Input: part model. Units: mm. Frame: model coordinates. A direction names the side the tool comes from. Give positions to 0.01 mm unless a question says otherwise; leave off trailing zeros. Write each loop counter-clockwise with the first axis right and the second up, starting at its lowest first coordinate (ties: lowest second). Pieces come first, ordered by that corner, then holes. Notation, with made-up numbers: (71.5, -30.5) -> (128.5, -30.5) arc R22 ccw to (128.5, -9.5) -> close; hole circle Ø6 at (-36.75, 5). An arc over 180 degrees is marked (long way). Answer as a JSON object with one key per item and string values. Group by question number.
from build123d import *

# Parameters (mm, degrees)
F0_R     = 0.8
F0_R_2   = 1.6
F0_R_3   = 1.2
F1_DEPTH = 4
F2_W     = 34.4678
F2_H     = 0.2
F3_DEPTH = 3.8


with BuildPart() as f1:
    # F0 (on Front) → F1 (new body)
    with BuildSketch(Plane.XZ):
        with BuildLine():
            Line((-76.973173, -27.461596), (-105.598973, -27.461596))
            ThreePointArc((-105.598973, -27.461596), (-107.664432, -28.317137), (-108.519973, -30.382596))
            Line((-108.519973, -30.382596), (-108.519973, -48.797596))
            ThreePointArc((-108.519973, -48.797596), (-107.664432, -50.863055), (-105.598973, -51.718596))
            Line((-105.598973, -51.718596), (-76.973173, -51.718596))
            ThreePointArc((-76.973173, -51.718596), (-74.907714, -50.863055), (-74.052173, -48.797596))
            Line((-74.052173, -48.797596), (-74.052173, -30.382596))
            ThreePointArc((-74.052173, -30.382596), (-74.907714, -28.317137), (-76.973173, -27.461596))
        make_face()
        with Locations((-102.017573, -45.266996)):
            Circle(F0_R, mode=Mode.SUBTRACT)
        with Locations((-97.648773, -45.266996)):
            Circle(F0_R, mode=Mode.SUBTRACT)
        with Locations((-93.279973, -45.266996)):
            Circle(F0_R, mode=Mode.SUBTRACT)
        with Locations((-99.833173, -41.482396)):
            Circle(F0_R, mode=Mode.SUBTRACT)
        with Locations((-95.464373, -41.482396)):
            Circle(F0_R, mode=Mode.SUBTRACT)
        with BuildLine():
            ThreePointArc((-77.666642, -47.210096), (-76.839663, -45.530643), (-75.379473, -46.702096))
            ThreePointArc((-75.379473, -46.702096), (-75.40802, -46.962285), (-75.492304, -47.210096))
            ThreePointArc((-75.492304, -47.210096), (-75.40802, -47.457906), (-75.379473, -47.718096))
            ThreePointArc((-75.379473, -47.718096), (-76.839663, -48.889548), (-77.666642, -47.210096))
        make_face(mode=Mode.SUBTRACT)
        with Locations((-88.911173, -45.266996)):
            Circle(F0_R, mode=Mode.SUBTRACT)
        with Locations((-91.095573, -41.482396)):
            Circle(F0_R, mode=Mode.SUBTRACT)
        with Locations((-86.726773, -41.482396)):
            Circle(F0_R, mode=Mode.SUBTRACT)
        with Locations((-76.579473, -39.590096)):
            Circle(F0_R_2, mode=Mode.SUBTRACT)
        with Locations((-102.017573, -37.697796)):
            Circle(F0_R, mode=Mode.SUBTRACT)
        with Locations((-97.648773, -37.697796)):
            Circle(F0_R, mode=Mode.SUBTRACT)
        with Locations((-93.279973, -37.697796)):
            Circle(F0_R, mode=Mode.SUBTRACT)
        with Locations((-99.833173, -33.913196)):
            Circle(F0_R, mode=Mode.SUBTRACT)
        with Locations((-95.464373, -33.913196)):
            Circle(F0_R, mode=Mode.SUBTRACT)
        with Locations((-88.911173, -37.697796)):
            Circle(F0_R, mode=Mode.SUBTRACT)
        with Locations((-91.095573, -33.913196)):
            Circle(F0_R, mode=Mode.SUBTRACT)
        with Locations((-86.726773, -33.913196)):
            Circle(F0_R, mode=Mode.SUBTRACT)
        with Locations((-76.579473, -31.970096)):
            Circle(F0_R_3, mode=Mode.SUBTRACT)
    extrude(amount=F1_DEPTH)

    # F2 (on face) → F3 (cut)
    with BuildSketch(Plane.XZ.offset(4)):
        with Locations((-91.286073, -33.913196)):
            Rectangle(F2_W, F2_H)
        with Locations((-91.286073, -37.697796)):
            Rectangle(F2_W, F2_H)
    extrude(amount=-F3_DEPTH, mode=Mode.SUBTRACT)


solid = f1.part
1. Section C-C (y = -1). State how many separate pieces and enclosed holes the cut face has, plus the area to 3 significant figures.
2. Contact query for a flat-ended pin moving along its axis: pin 1 Ø1.4 at (x, z) = (-91.1, -33.91) entering from -Y. Output: stop coordinate, or through.
3. Mould query, pull axis Z, two halves, no side actions, for faces 3 (the face through (-92, -4, -36)), 4 (the face through (-91, -2, -27.462)), 5 (the face through (-99.094, -1.972, -34.22)), 6 (the face through (-89.55, -1.97, -45.75)). Classes: pulls with the +Z half, pulls with the -Z half, needs draft (parallel to the pull), parting line crosses it, or undercut.
4. Section D-D (x = -93.5). Return the cut outline in (y, z).
5. Section A-A (x = -102). Return the cut outline in (y, z), plus the area to 3 significant figures.
6. Reachability of faces 1 (the face through (-92.54, -1.97, -38)), 2 (the face through (-95, -2, -37.598)) from +Z, -Z, +X, -X, +Y, -Y: full face, straight path, thin tool, end or side. Return the list, or none.
7. Line query: line 1 (Z direction, x = -103.5, y = -1.7); line 2 (Z direction, x = -95, y = -0.25); line 3 (Z direction, x = -97, y = -2.35). Output: solid intervals per line, ascending.
8. Section B-B (x = -81). Return the cut outline in (y, z), plus the area to 3 significant figures.
Working result:
{
 "1": {"separate pieces": "3", "enclosed holes": "11", "area": "766 mm^2"},
 "2": {"pin 1": "passes through"},
 "3": {"face 3": "needs draft", "face 4": "pulls with the +Z half", "face 5": "undercut", "face 6": "undercut"},
 "4": {"outline": "(-4, -51.72) -> (0, -51.72) -> (0, -46.04) -> (-4, -46.04) -> close; (-4, -44.5) -> (0, -44.5) -> (0, -38.47) -> (-4, -38.47) -> close; (-4, -36.93) -> (0, -36.93) -> (0, -27.46) -> (-4, -27.46) -> (-4, -33.81) -> (-0.2, -33.81) -> (-0.2, -34.01) -> (-4, -34.01) -> close"},
 "5": {"outline": "(-4, -51.72) -> (0, -51.72) -> (0, -46.07) -> (-4, -46.07) -> close; (-4, -44.47) -> (0, -44.47) -> (0, -38.5) -> (-4, -38.5) -> close; (-4, -36.9) -> (0, -36.9) -> (0, -27.46) -> (-4, -27.46) -> (-4, -33.81) -> (-0.2, -33.81) -> (-0.2, -34.01) -> (-4, -34.01) -> close", "area": "83.5 mm^2"},
 "6": {"face 1": "+Y, -Y", "face 2": "+X, -X, -Y"},
 "7": {"line 1": "z = -51.72 to -37.8, -37.6 to -34.01, -33.81 to -27.46", "line 2": "z = -51.72 to -42.13, -40.83 to -37.8, -37.6 to -34.56, -33.26 to -27.46", "line 3": "z = -51.72 to -45.74, -44.8 to -38.17, -37.23 to -34.01, -33.81 to -27.46"},
 "8": {"outline": "(-4, -51.72) -> (0, -51.72) -> (0, -27.46) -> (-4, -27.46) -> (-4, -33.81) -> (-0.2, -33.81) -> (-0.2, -34.01) -> (-4, -34.01) -> (-4, -37.6) -> (-0.2, -37.6) -> (-0.2, -37.8) -> (-4, -37.8) -> close", "area": "95.5 mm^2"}
}
